```python
from build123d import *

# Parameters (mm, degrees)
SKETCH1_W           = 25
SKETCH1_H           = 211.5
BOSS_EXTRUDE1_DEPTH = 10
SKETCH2_W           = 10
SKETCH2_H           = 15
SKETCH2_H_2         = 10
SKETCH2_W_2         = 191.5
BOSS_EXTRUDE2_DEPTH = 45
SKETCH3_W           = 185
SKETCH3_H           = 3.5
CUT_EXTRUDE1_DEPTH  = 10
SKETCH4_R           = 1.9
CUT_EXTRUDE2_DEPTH  = 220.959655392
SKETCH5_R           = 3.35
CUT_EXTRUDE3_DEPTH  = 2.5
CUT_EXTRUDE4_DEPTH  = 2.5
LPATTERN1_COUNT     = 3
LPATTERN1_PITCH     = 88.5
CUT_EXTRUDE5_REACH  = 224.671
BOSS_EXTRUDE4_REACH = 224.671
CUT_EXTRUDE6_REACH  = 224.671
SKETCH11_W          = 78.5
SKETCH11_H          = 0.625
SKETCH11_W_2        = 113
SKETCH12_W          = 3.5
SKETCH12_H          = 34
CUT_EXTRUDE8_DEPTH  = 5
CUT_EXTRUDE9_DEPTH  = 5
SKETCH14_W          = 78.5
SKETCH14_H          = 5
CUT_EXTRUDE10_DEPTH = 14.375
CUT_EXTRUDE11_REACH = 224.671
SKETCH15_R          = 1.9
CUT_EXTRUDE12_DEPTH = 2.5
LPATTERN2_COUNT     = 2
LPATTERN2_PITCH     = 64


with BuildPart() as part:
    # Sketch1 → Boss-Extrude1 (new body)
    with BuildSketch(Plane(origin=(0, 0, 0), x_dir=(0, 1, 0), z_dir=(0, 0, 1))):
        with Locations((12.5, 105.75)):
            Rectangle(SKETCH1_W, SKETCH1_H)
    boss_extrude1 = extrude(amount=BOSS_EXTRUDE1_DEPTH)

    # Sketch2 → Boss-Extrude2 (add)
    with BuildSketch(Plane.XY.offset(10)):
        with Locations((-5, 17.5)):
            Rectangle(SKETCH2_W, SKETCH2_H)
        with Locations((-5, 5)):
            Rectangle(SKETCH2_W, SKETCH2_H_2)
        with Locations((-105.75, 5)):
            Rectangle(SKETCH2_W_2, SKETCH2_H_2)
        with Locations((-206.5, 5)):
            Rectangle(SKETCH2_W, SKETCH2_H_2)
        with Locations((-206.5, 17.5)):
            Rectangle(SKETCH2_W, SKETCH2_H)
    extrude(amount=BOSS_EXTRUDE2_DEPTH)

    # Mirror1: Boss-Extrude1 across plane
    add(boss_extrude1.mirror(Plane.XY.offset(32.5)))

    # Sketch3 → Cut-Extrude1 (cut)
    with BuildSketch(Plane(origin=(0, 25, 0), x_dir=(-1, 0, 0), z_dir=(0, 1, 0))):
        with Locations((105.75, 5)):
            Rectangle(SKETCH3_W, SKETCH3_H)
    extrude(amount=-CUT_EXTRUDE1_DEPTH, mode=Mode.SUBTRACT)

    # Sketch4 → Cut-Extrude2 (cut, through all)
    with BuildSketch(Plane(origin=(0, 0, 10), x_dir=(-1, 0, 0), z_dir=(0, 0, 1))):
        with Locations(Location((194.25, -20, 0), (0, 0, 180))):
            Circle(SKETCH4_R)
    cut_extrude2 = extrude(amount=-CUT_EXTRUDE2_DEPTH, mode=Mode.SUBTRACT)

    # Sketch5 → Cut-Extrude3 (cut)
    with BuildSketch(Plane(origin=(0, 0, 0), x_dir=(1, 0, 0), z_dir=(0, 0, -1))):
        with Locations(Location((-194.25, -20, 0), (0, 0, 180))):
            Circle(SKETCH5_R)
    cut_extrude3 = extrude(amount=-CUT_EXTRUDE3_DEPTH, mode=Mode.SUBTRACT)

    # Sketch6 → Cut-Extrude4 (cut)
    with BuildSketch(Plane.XY.offset(10)):
        Polygon((-192.297927406, 23.381088913), (-196.202072594, 23.381088913), (-198.154145188, 20), (-196.202072594, 16.618911087), (-192.297927406, 16.618911087), (-190.345854812, 20), align=None)
    cut_extrude4 = extrude(amount=-CUT_EXTRUDE4_DEPTH, mode=Mode.SUBTRACT)

    # LPattern1: Cut-Extrude2, Cut-Extrude3, Cut-Extrude4 ×3
    with Locations(*[(i * LPATTERN1_PITCH, 0, 0) for i in range(1, LPATTERN1_COUNT)]):
        add(cut_extrude2, mode=Mode.SUBTRACT)
        add(cut_extrude3, mode=Mode.SUBTRACT)
        add(cut_extrude4, mode=Mode.SUBTRACT)

    # Sketch9 → Cut-Extrude5 (cut, up to next)
    with BuildSketch(Plane.XZ, mode=Mode.PRIVATE) as cut_extrude5_sk1:
        Polygon((-10, 39), (0, 39), (0, 65), (-123, 65), align=None)
    cut_extrude5_tool1 = extrude(cut_extrude5_sk1.sketch, amount=-CUT_EXTRUDE5_REACH, mode=Mode.PRIVATE) & part.part
    add(cut_extrude5_tool1.solids().sort_by_distance((-41.250627, 0, 55.681704))[0], mode=Mode.SUBTRACT)

    # Sketch10 → Boss-Extrude4 (add, up to next)
    with BuildSketch(Plane(origin=(0, 25, 0), x_dir=(-1, 0, 0), z_dir=(0, 1, 0)), mode=Mode.PRIVATE) as boss_extrude4_sk1:
        Polygon((123, 65), (10, 39), (10, 29), (123, 55), align=None)
    boss_extrude4_tool1 = extrude(boss_extrude4_sk1.sketch, amount=-BOSS_EXTRUDE4_REACH, mode=Mode.PRIVATE) - part.part
    add(boss_extrude4_tool1.solids().sort_by_distance((-66.5, 25, 47))[0])

    # Sketch11 → Cut-Extrude6 (cut, up to next)
    with BuildSketch(Plane.XY.offset(65), mode=Mode.PRIVATE) as cut_extrude6_sk1:
        with Locations((-162.25, 24.6875)):
            Rectangle(SKETCH11_W, SKETCH11_H)
    cut_extrude6_tool1 = extrude(cut_extrude6_sk1.sketch, amount=-CUT_EXTRUDE6_REACH, mode=Mode.PRIVATE) & part.part
    # Sketch11 → Cut-Extrude6 (cut, up to next)
    with BuildSketch(Plane.XY.offset(65), mode=Mode.PRIVATE) as cut_extrude6_sk2:
        with Locations((-66.5, 24.6875)):
            Rectangle(SKETCH11_W_2, SKETCH11_H)
    cut_extrude6_tool2 = extrude(cut_extrude6_sk2.sketch, amount=-CUT_EXTRUDE6_REACH, mode=Mode.PRIVATE) & part.part
    add(cut_extrude6_tool1.solids().sort_by_distance((-162.25, 24.6875, 65))[0], mode=Mode.SUBTRACT)
    add(cut_extrude6_tool2.solids().sort_by_distance((-66.5, 24.6875, 65))[0], mode=Mode.SUBTRACT)

    # Sketch12 → Cut-Extrude8 (cut)
    with BuildSketch(Plane(origin=(0, 25, 0), x_dir=(-1, 0, 0), z_dir=(0, 1, 0))):
        with Locations((5, 22)):
            Rectangle(SKETCH12_W, SKETCH12_H)
    extrude(amount=-CUT_EXTRUDE8_DEPTH, mode=Mode.SUBTRACT)

    # Sketch13 → Cut-Extrude9 (cut)
    with BuildSketch(Plane(origin=(0, 25, 0), x_dir=(-1, 0, 0), z_dir=(0, 1, 0))):
        Polygon((204.75, 15), (204.75, 5), (208.25, 5), (208.25, 15), (208.25, 65), (204.75, 65), align=None)
    extrude(amount=-CUT_EXTRUDE9_DEPTH, mode=Mode.SUBTRACT)

    # Sketch14 → Cut-Extrude10 (cut)
    with BuildSketch(Plane(origin=(0, 24.375, 0), x_dir=(-1, 0, 0), z_dir=(0, 1, 0))):
        with Locations((162.25, 57.5)):
            Rectangle(SKETCH14_W, SKETCH14_H)
    extrude(amount=-CUT_EXTRUDE10_DEPTH, mode=Mode.SUBTRACT)

    # Sketch15 → Cut-Extrude11 (cut, up to next)
    with BuildSketch(Plane.XY.offset(65), mode=Mode.PRIVATE) as cut_extrude11_sk1:
        with Locations((-194.25, 19.375)):
            Circle(SKETCH15_R)
    cut_extrude11_tool1 = extrude(cut_extrude11_sk1.sketch, amount=-CUT_EXTRUDE11_REACH, mode=Mode.PRIVATE) & part.part
    cut_extrude11 = cut_extrude11_tool1.solids().sort_by_distance((-194.25, 19.375, 65))[0]
    add(cut_extrude11, mode=Mode.SUBTRACT)

    # Sketch16 → Cut-Extrude12 (cut)
    with BuildSketch(Plane(origin=(0, 0, 60), x_dir=(1, 0, 0), z_dir=(0, 0, -1))):
        Polygon((-192.297927406, -15.993911087), (-196.202072594, -15.993911087), (-198.154145188, -19.375), (-196.202072594, -22.756088913), (-192.297927406, -22.756088913), (-190.345854812, -19.375), align=None)
    cut_extrude12 = extrude(amount=-CUT_EXTRUDE12_DEPTH, mode=Mode.SUBTRACT)

    # LPattern2: Cut-Extrude11, Cut-Extrude12 ×2
    with Locations(*[(i * LPATTERN2_PITCH, 0, 0) for i in range(1, LPATTERN2_COUNT)]):
        add(cut_extrude11, mode=Mode.SUBTRACT)
        add(cut_extrude12, mode=Mode.SUBTRACT)


solid = part.part
```
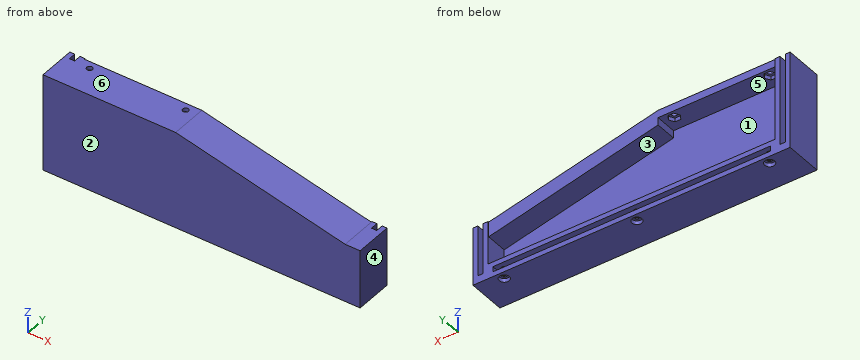
Design review of the part built by this model. Coordinates are the model's own, in mm. Face numbers are marked on the shaded views. A direction names the side the tool comes from. Give positions to 0.01 mm unless a question says otherwise; leave off trailing zeros. Order: outer loops, then holes, each group sorted by start corner. A loop starts at its lowest first (then second) coordinate and runs counter-clockwise, first axis right, second up. Notation, with made-up numbers: (23.5, 84.5) - (81.5, 84.5) arc R14 ccw to (81.5, 99.5) - close; hole circle Ø8 at (-1, 63). An arc over 180 degrees is marked (long way). Use a Markdown table: item, result. Add a question column.
(1) Wall thickness on probe 1 along Z at (x, y) = (-192, 20); probe 2 along X at (y, z) = (13, 21); probe 3 along Z at (x, y) = (-45.5, 16.5): over which ranges is each line inside the solid? List them lowest first. Write a range as [from, to].
(2) Mouldability with a two-part tool opening along X and no side actions: class the marked faces 1, 2, 3 and 4 as +X half, -X half, draft (parallel to the pull), parting line (faces both ways), or undercut.
(3) Clearance check with flat-ended pins moving along their axes: P1, Ø2, axis at x = -18.5, y = 19, coming from the -Z side; P2, Ø1.2, axis at x = -130, z = 61.5, coming from the +Y side (3 decimals); P3, Ø1, axis at x = -47.5, y = 10.5, coming from the +Z side. State where each tip first meets the part, or that it passes through.
(4) Add section C-C on z = 12.5. Give the boundary of the cut face in (x, y).
(5) Machinability: for the marked faces 5 and 6, which of the approach directions +Z, -Z, +X, -X, +Y, -Y give a long, thin tool a straight path to every point of the face, cutting with its end or side? Answer none if there is none.
(6) Add section D-D on x = -184. Give the boundary of the cut face in (y, z) (3 decimals).
(7) Add section B-B on y = 13. Give the boundary of the cut face in (x, z).
(8) Add section A-A on x = -130.25. Give the boundary of the cut face in (y, z) (3 decimals), then the cut area to 3 significant figures.
Report:
| question | item | result |
|---|---|---|
| 1 | probe 1 | z = [2.5, 3.25], [6.75, 7.5], [62.5, 65] |
| 1 | probe 2 | x = [-211.5, -201.5], [-10, 0] |
| 1 | probe 3 | z = [0, 3.25], [6.75, 10], [37.17, 47.17] |
| 2 | face 1 | undercut |
| 2 | face 2 | draft |
| 2 | face 3 | undercut |
| 2 | face 4 | +X half |
| 3 | P1 | stops at z = 2.5 |
| 3 | P2 | stops at y = 24.375 |
| 3 | P3 | stops at z = 47.74 |
| 4 | outline | (-211.5, 0) - (0, 0) - (0, 25) - (-3.25, 25) - (-3.25, 20) - (-6.75, 20) - (-6.75, 25) - (-10, 25) - (-10, 10) - (-201.5, 10) - (-201.5, 25) - (-204.75, 25) - (-204.75, 20) - (-208.25, 20) - (-208.25, 25) - (-211.5, 25) - close |
| 5 | face 5 | +Y |
| 5 | face 6 | +Z, +X, -X, +Y, -Y |
| 6 | outline | (0, 0) - (25, 0) - (25, 3.25) - (15, 3.25) - (15, 6.75) - (25, 6.75) - (25, 10) - (10, 10) - (10, 60) - (24.375, 60) - (24.375, 65) - (0, 65) - close |
| 7 | outline | (-211.5, 0) - (0, 0) - (0, 39) - (-10, 39) - (-123, 65) - (-211.5, 65) - close; hole (-201.5, 10) - (-10, 10) - (-10, 29) - (-123, 55) - (-123, 60) - (-201.5, 60) - close |
| 8 | outline | (0, 0) - (25, 0) - (25, 3.25) - (15, 3.25) - (15, 6.75) - (25, 6.75) - (25, 10) - (10, 10) - (10, 60) - (15.994, 60) - (15.994, 62.5) - (17.475, 62.5) - (17.475, 65) - (0, 65) - close; (21.275, 62.5) - (22.756, 62.5) - (22.756, 60) - (24.375, 60) - (24.375, 65) - (21.275, 65) - close |
| 8 | area | 810 mm² |
